Work out the finished part from the listing and answer in its coordinate system (mm). A direction names the side the tool comes from. Give positions to 0.01 mm unless a question says otherwise; leave off trailing zeros. Loops run counter-clockwise (first coordinate to the right, second up) from the corner with the lowest first, then second, coordinate; pieces in that order, holes last.
from build123d import *

# Parameters (mm, degrees)
SKETCH1_R           = 19.05
SKETCH1_R_2         = 2.75
BOSS_EXTRUDE1_DEPTH = 5
CUT_EXTRUDE1_DEPTH  = 4.1
SKETCH5_W           = 12.6
SKETCH5_H           = 22.5
BOSS_EXTRUDE2_DEPTH = 5
SKETCH6_R           = 0.75
CUT_EXTRUDE2_DEPTH  = 5
CUT_EXTRUDE3_DEPTH  = 5


with BuildPart() as part:
    # Sketch1 → Boss-Extrude1 (new body)
    with BuildSketch(Plane(origin=(0, 0, 0), x_dir=(1, 0, 0), z_dir=(0, 1, 0))):
        Circle(SKETCH1_R)
        Circle(SKETCH1_R_2, mode=Mode.SUBTRACT)
    extrude(amount=BOSS_EXTRUDE1_DEPTH)

    # Sketch4 → Cut-Extrude1 (cut)
    with BuildSketch(Plane(origin=(0, 0, 0), x_dir=(1, 0, 0), z_dir=(0, 1, 0))):
        Polygon((0, 4.641896164), (-4.02, 2.320948082), (-4.02, -2.320948082), (0, -4.641896164), (4.02, -2.320948082), (4.02, 2.320948082), align=None)
    extrude(amount=CUT_EXTRUDE1_DEPTH, mode=Mode.SUBTRACT)

    # Sketch5 → Boss-Extrude2 (add)
    with BuildSketch(Plane.ZY.offset(10.98)):
        with BuildLine():
            Line((-12, 5), (12, 5))
            Line((12, 5), (9.265979265, 36.25))
            ThreePointArc((9.265979265, 36.25), (0, 44.740705658), (-9.265979265, 36.25))
            Line((-9.265979265, 36.25), (-12, 5))
        make_face()
        with Locations((0, 25)):
            Rectangle(SKETCH5_W, SKETCH5_H, mode=Mode.SUBTRACT)
    boss_extrude2 = extrude(amount=-BOSS_EXTRUDE2_DEPTH)

    # Mirror1: Boss-Extrude2 across plane
    add(boss_extrude2.mirror(Plane(origin=(0, 0, 0), x_dir=(0, 0, 1), z_dir=(1, 0, 0))))

    # Sketch6 → Cut-Extrude2 (cut)
    with BuildSketch(Plane.ZY.offset(10.98)):
        with Locations((0, 38.715999834)):
            Circle(SKETCH6_R)
        with Locations((0, 11.284000166)):
            Circle(SKETCH6_R)
    extrude(amount=-CUT_EXTRUDE2_DEPTH, mode=Mode.SUBTRACT)

    # Sketch7 → Cut-Extrude3 (cut)
    with BuildSketch(Plane.ZY.offset(-5.98)):
        with BuildLine():
            Line((-4.490705658, 36.25), (4.490705658, 36.25))
            ThreePointArc((4.490705658, 36.25), (0, 40.740705658), (-4.490705658, 36.25))
        make_face()
    extrude(amount=-CUT_EXTRUDE3_DEPTH, mode=Mode.SUBTRACT)


solid = part.part
Item 1: Find section C-C, the plane y = 3.5. Write down the section's boundary in (x, z), plus the area to 3 significant figures.
Item 2: Find section B-B, the plane z = 3.5. Write down the section's boundary in (x, y).
Item 3: Consider line 1 (Y direction, x = -9.15, z = 0); line 2 (X direction, y = 4.45, z = 0); line 3 (X direction, y = 12.5, z = 3.5). Determine where each line is inside the solid, lowest interval first.
Item 4: Find section A-A, the plane y = 15. Write down the section's boundary in (x, z).
Item 5: Determine the mould class of faces 1 (the face through (4, 5, 0)), 2 (the face through (0, 0, -5)), 3 (the face through (2.038, 2.021, -3.465)), 4 (the face through (-9, 36.25, 0)) for opening direction Y: released by +Y, released by -Y, zero draft, split by the parting line, or undercut.
Item 6: Find section D-D, the plane x = 14. Write down the section's boundary in (y, z), plus the area to 3 significant figures.
Item 7: For faces 5 (the face through (5.98, 21, 8)), 6 (the face through (9, 13.75, 0)), 7 (the face through (4.02, 2, 0)), 8 (the face through (-8.52, 20.41, 10.65)), determine the directions among +Z, -Z, +X, -X, +Y, -Y from which every point of the face is accessible in a straight line to the end or side of a thin tool.
Item 8: Flat-ended cylindrical pins translate along their axes: pin 1 Ø4 at (x, y) = (8.5, 26.5) entering from -Z; pin 2 Ø7 at (y, z) = (30, -3.5) entering from +X; pin 3 Ø5.5 at (x, y) = (9, 23) entering from +Z. Find the tip coordinate at first contact, or state that the pin passes through.
Ans:
1. outline: circle Ø38.1 at (0, 0); hole (-4.02, -2.32) - (0, -4.64) - (4.02, -2.32) - (4.02, 2.32) - (0, 4.64) - (-4.02, 2.32) - close
1. area: 1,080 mm2
2. outline: (-18.73, 0) - (-1.98, 0) - (-1.98, 4.1) - (1.98, 4.1) - (1.98, 0) - (18.73, 0) - (18.73, 5) - (10.98, 5) - (10.98, 13.75) - (5.98, 13.75) - (5.98, 5) - (-5.98, 5) - (-5.98, 13.75) - (-10.98, 13.75) - (-10.98, 5) - (-18.73, 5) - close; (-10.98, 36.25) - (-5.98, 36.25) - (-5.98, 44.06) - (-10.98, 44.06) - close; (5.98, 39.06) - (10.98, 39.06) - (10.98, 44.06) - (5.98, 44.06) - close
3. line 1: y = 0 to 10.53, 12.03 to 13.75, 36.25 to 37.97, 39.47 to 44.74
3. line 2: x = -19.05 to -2.75, 2.75 to 19.05
3. line 3: x = -10.98 to -5.98, 5.98 to 10.98
4. outline: (-10.98, -11.13) - (-5.98, -11.13) - (-5.98, -6.3) - (-10.98, -6.3) - close; (-10.98, 6.3) - (-5.98, 6.3) - (-5.98, 11.13) - (-10.98, 11.13) - close; (5.98, -11.13) - (10.98, -11.13) - (10.98, -6.3) - (5.98, -6.3) - close; (5.98, 6.3) - (10.98, 6.3) - (10.98, 11.13) - (5.98, 11.13) - close
5. face 1: released by +Y
5. face 2: released by -Y
5. face 3: zero draft
5. face 4: undercut
6. outline: (0, -12.92) - (5, -12.92) - (5, 12.92) - (0, 12.92) - close
6. area: 129 mm2
7. face 5: +Z, -Z, +Y
7. face 6: +X, -X
7. face 7: -Y
7. face 8: +Z, +X, -X, +Y
8. pin 1: stops at z = -10.29
8. pin 2: stops at x = 10.98
8. pin 3: stops at z = 10.67
